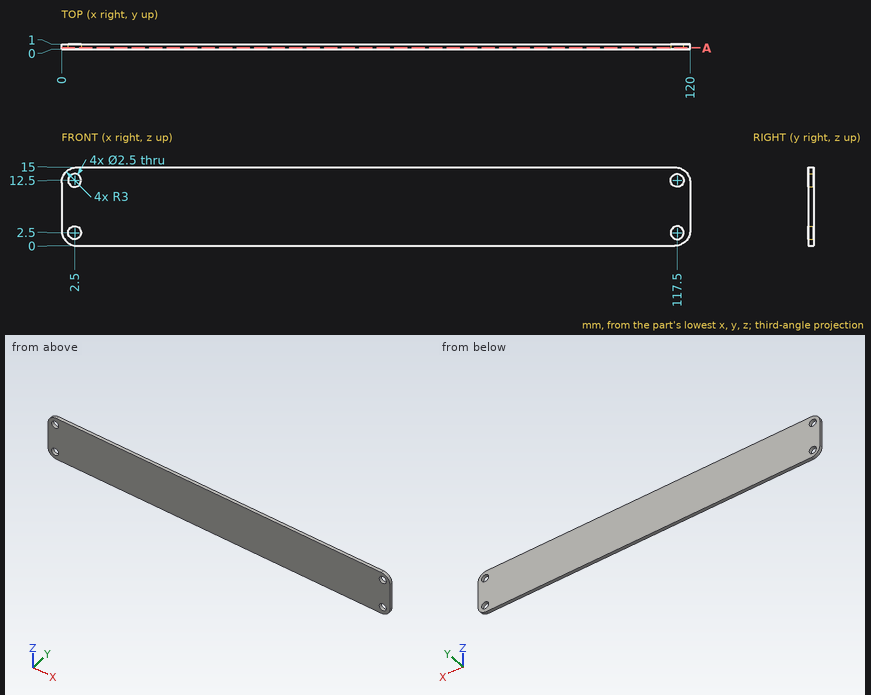
Geometry: see drawing. Coordinates: mm, zero at the bounding-box minimum. Give positions to 0.01 mm unless a question says otherwise; leave off trailing zeros. Write each loop counter-clockwise with the first axis right and the second up, starting at its lowest first coordinate (ties: lowest second). Pieces come first, ordered by that corner, then holes. Notation, with made-up numbers: M 40,68.25 L 83,68.25 A27 ccw 83,99.25 Z; hole C -9.75,-33.75 d3. An arc over 180 degrees is marked long. Answer as a JSON object with one key per item and string values.
Q1. Ray query, line 1 along Z through (x, y) = (117.5, 0.7); line 2 along X through (y, z) = (0.6, 1.75); line 3 along X through (y, z) = (0.3, 12.25). Return the intervals inside material, ascending.
Geometry check:
{"line 1": "z = 0.04 to 1.25, 3.75 to 11.25, 13.75 to 14.96", "line 2": "x = 0.27 to 1.5, 3.5 to 116.5, 118.5 to 119.73", "line 3": "x = 0.01 to 1.28, 3.72 to 116.28, 118.72 to 119.99"}
Q2. Cut plane A-A, the plane y = 0.25. Return the cut outline in (x, z), then the cut area to 3 significant figures.
Geometry check:
{"outline": "M 0,3 A3 ccw 3,0 L 117,0 A3 ccw 120,3 L 120,12 A3 ccw 117,15 L 3,15 A3 ccw 0,12 Z; hole C 2.5,2.5 d2.5; hole C 2.5,12.5 d2.5; hole C 117.5,2.5 d2.5; hole C 117.5,12.5 d2.5", "area": "1,770 mm^2"}
Q3. Contact query for flat-ended pins moving along their axis: P1, Ø3, axis at x = 117.5, z = 2.5, coming from the +Y side; P2, Ø1.5, axis at x = 2.5, z = 2.5, coming from the -Y side. Output: stop coordinate, or through.
Geometry check:
{"P1": "stops at y = 1", "P2": "passes through"}
